from build123d import *

# Parameters (mm, degrees)
F0_W     = 111.9791269302
F0_H     = 211.9790837169
F1_DEPTH = 52.578
F0_W_2   = 50.8
F0_H_2   = 50.8
F0_W_3   = 47.3935049959
F0_H_3   = 47.4935397506
F2_DEPTH = 52.832
F3_W     = 48.1118559837
F3_H     = 149.3962490931
F4_DEPTH = 53.594
F5_W     = 111.9791269302
F5_H     = 211.9790837169
F6_DEPTH = 2.54
F7_R     = 2.6479987439
F8_DEPTH = 48.006


with BuildPart() as f1:
    # F0 (on Front) → F1 (new body)
    with BuildSketch(Plane.XZ):
        with Locations((0.8473545313, 47.6342774928)):
            Rectangle(F0_W, F0_H)
        Polygon((-50.0439400733, 97.9935325928), (-50.0439400733, 148.7935325928), (0.7560599267, 148.7935325928), (51.5560599267, 148.7935325928), (51.5560599267, 97.9935325928), (51.5560599267, 47.1935325928), (51.5560599267, -3.6064674072), (51.5560599267, -54.4064674072), (0.7560599267, -54.4064674072), (-50.0439400733, -54.4064674072), align=None, mode=Mode.SUBTRACT)
    extrude(amount=F1_DEPTH)

    # F0 (on Front) → F2 (join)
    with BuildSketch(Plane.XZ):
        with Locations((-24.6439400733, 123.3935325928)):
            Rectangle(F0_W_2, F0_H_2)
        with Locations((-24.4151034858, 123.106200248)):
            Rectangle(F0_W_3, F0_H_3, mode=Mode.SUBTRACT)
        with Locations((26.1560599267, 123.3935325928)):
            Rectangle(F0_W_2, F0_H_2)
        with Locations((26.312828064, 123.2058629394)):
            Rectangle(F0_W_3, F0_H_3, mode=Mode.SUBTRACT)
        with Locations((26.1560599267, 72.5935325928)):
            Rectangle(F0_W_2, F0_H_2)
        with Locations((26.148814708, 72.9721300304)):
            Rectangle(F0_W_3, F0_H_3, mode=Mode.SUBTRACT)
        Polygon((0.7560599267, 97.9935325928), (-50.0439400733, 97.9935325928), (-50.0439400733, -54.4064674072), (0.7560599267, -54.4064674072), (0.7560599267, -3.6064674072), (0.7560599267, 47.1935325928), align=None)
        with Locations((26.1560599267, 21.7935325928)):
            Rectangle(F0_W_2, F0_H_2)
        with Locations((26.2633450329, 21.912215976)):
            Rectangle(F0_W_3, F0_H_3, mode=Mode.SUBTRACT)
        with Locations((26.1560599267, -29.0064674072)):
            Rectangle(F0_W_2, F0_H_2)
        with Locations((26.0739140213, -29.1093634441)):
            Rectangle(F0_W_3, F0_H_3, mode=Mode.SUBTRACT)
    extrude(amount=F2_DEPTH)

    # F3 (on face) → F4 (cut)
    with BuildSketch(Plane.XZ.offset(52.832)):
        with Locations((-24.0559279919, 21.8419912271)):
            Rectangle(F3_W, F3_H)
    extrude(amount=-F4_DEPTH, mode=Mode.SUBTRACT)

    # F5 (on face) → F6 (join)
    with BuildSketch(Plane(origin=(0, 0, 0), x_dir=(-1, 0, 0), z_dir=(0, 1, 0))):
        with Locations((-0.8473545313, 47.6342774928)):
            Rectangle(F5_W, F5_H)
    extrude(amount=F6_DEPTH)

    # F7 (on face) → F8 (join)
    with BuildSketch(Plane(origin=(0, 0, 0), x_dir=(0, -1, 0), z_dir=(-1, 0, 0))):
        with Locations((24.5460756123, 87.587043643)):
            Circle(F7_R)
    extrude(amount=F8_DEPTH)


solid = f1.part
Build history of the part. All positions in model axes, mm. A direction names the side the tool comes from. Round coordinates to 2 decimals unless told otherwise and drop trailing zeros. Write each loop counter-clockwise with the first axis right and the second up, starting at its lowest first coordinate (ties: lowest second). Pieces come first, ordered by that corner, then holes. Notation, with made-up numbers: (20, 68.5) - (46, 68.5) arc R19 cw to (46, 86.5) - close; hole circle Ø11 at (55.5, 83). An arc over 180 degrees is marked (long way). Use CSV: the item, a comma, the result in double quotes.
(1) Band-saw the part on D-D (x = -10.5). Write the cut outline in (y, z), plus the area to 3 significant figures.
Response:
outline,"(-52.83, -54.41) - (-52.58, -54.41) - (-52.58, -58.36) - (2.54, -58.36) - (2.54, 153.62) - (-52.58, 153.62) - (-52.58, 148.79) - (-52.83, 148.79) - (-52.83, 146.85) - (0, 146.85) - (0, 99.36) - (-52.83, 99.36) - (-52.83, 96.54) - (0, 96.54) - (0, -52.86) - (-52.83, -52.86) - close; circle Ø5.3 at (-24.55, 87.59)"
area,"1,360 mm²"
(2) Band-saw the part on B-B (z = 62.5). Write the cut outline in (x, y).
Response:
outline,"(-55.14, -52.58) - (-50.04, -52.58) - (-50.04, -52.83) - (-48.11, -52.83) - (-48.11, 0) - (0, 0) - (0, -52.83) - (2.45, -52.83) - (2.45, 0) - (49.85, 0) - (49.85, -52.83) - (51.56, -52.83) - (51.56, -52.58) - (56.84, -52.58) - (56.84, 2.54) - (-55.14, 2.54) - close"
(3) Band-saw the part on A-A (y = -36). Write the cut outline in (x, z).
Response:
outline,"(-55.14, -58.36) - (56.84, -58.36) - (56.84, 153.62) - (-55.14, 153.62) - close; hole (-48.11, -52.86) - (0, -52.86) - (0, 96.54) - (-48.11, 96.54) - close; hole (-48.11, 99.36) - (-0.72, 99.36) - (-0.72, 146.85) - (-48.11, 146.85) - close; hole (2.38, -52.86) - (49.77, -52.86) - (49.77, -5.36) - (2.38, -5.36) - close; hole (2.45, 49.23) - (49.85, 49.23) - (49.85, 96.72) - (2.45, 96.72) - close; hole (2.57, -1.83) - (49.96, -1.83) - (49.96, 45.66) - (2.57, 45.66) - close; hole (2.62, 99.46) - (50.01, 99.46) - (50.01, 146.95) - (2.62, 146.95) - close"
(4) Wall check: line 1 (X direction, y = -16.5, z = 117); line 2 (X direction, y = -13, z = -38); line 3 (Z direction, x = -15, y = -47). Give the ranges that are in metal, low to high.
Response:
line 1,"-55.14 to -48.11, -0.72 to 2.62, 50.01 to 56.84"
line 2,"-55.14 to -48.11, 0 to 2.38, 49.77 to 56.84"
line 3,"-58.36 to -52.86, 96.54 to 99.36, 146.85 to 153.62"
(5) Band-saw the part on C-C (x = 45). Write the cut outline in (y, z), plus the area to 3 significant figures.
Response:
outline,"(-52.83, -54.41) - (-52.58, -54.41) - (-52.58, -58.36) - (2.54, -58.36) - (2.54, 153.62) - (-52.58, 153.62) - (-52.58, 148.79) - (-52.83, 148.79) - (-52.83, 146.95) - (0, 146.95) - (0, 99.46) - (-52.83, 99.46) - (-52.83, 96.72) - (0, 96.72) - (0, 49.23) - (-52.83, 49.23) - (-52.83, 45.66) - (0, 45.66) - (0, -1.83) - (-52.83, -1.83) - (-52.83, -5.36) - (0, -5.36) - (0, -52.86) - (-52.83, -52.86) - close"
area,"1,700 mm²"
(6) Pin check, flat tip, straight feed: P1, Ø23.5, axis at x = 36.5, z = 31.5, coming from the -Y side. Stop position of the tip, or through.
Response:
P1,"y = 0"
(7) 3-axis set-ups, long thin cutter, end or side, ignore diameter. For faces 1 (the flat face through (2, -25, -58.355)), 2 (the flat face through (-24, -27, 96.54)): which of +Z, -Z, +X, -X, +Y, -Y reach the whole face in a straight line?
Response:
face 1,"-Z, +X, -X, +Y, -Y"
face 2,"-Y"
